```python
from build123d import *

# Parameters (mm, degrees)
SKETCH005_W    = 252
SKETCH005_H    = 268
PAD005_DEPTH   = 60
FILLET003_R    = 8
THICKNESS001_T = -3


with BuildPart() as part:
    # Sketch005 → Pad005 (new body)
    with BuildSketch(Plane.XY):
        with Locations((0, -134)):
            Rectangle(SKETCH005_W, SKETCH005_H)
    extrude(amount=PAD005_DEPTH)

    # Fillet003
    fillet003_edges = [part.edges().sort_by_distance(p)[0] for p in [
        (126, -268, 30),
        (-126, -268, 30),
    ]]
    fillet(fillet003_edges, radius=FILLET003_R)

    # Thickness001
    thickness001_openings = [part.faces().sort_by_distance(p)[0] for p in [
        (0, -133.946203, 60),
        (0, 0, 30),
        (0, -133.946203, 0),
    ]]
    offset(amount=THICKNESS001_T, openings=thickness001_openings)


solid = part.part
```
Input: part model. Units: mm. Frame: model coordinates. A direction names the side the tool comes from. Round coordinates to 2 decimals unless told otherwise and drop trailing zeros. Loops run counter-clockwise (first coordinate to the right, second up) from the corner with the lowest first, then second, coordinate; pieces in that order, holes last.
1) Section query C-C on x = -54.5. Return the cut outline in (y, z), plus the area to 3 significant figures.
Ans:
outline: (-268, 0) - (-265, 0) - (-265, 60) - (-268, 60) - close
area: 180 mm2
2) Material intervals for line 1 (X direction, y = -61, z = 19); line 2 (Y direction, x = -108, z = 42), sorted ascending.
Ans:
line 1: x = -126 to -123, 123 to 126
line 2: y = -268 to -265
3) Pin query (flat end, axial travel): pin 1 (8 mm diameter, centred on x = 89.5, z = 22, fed in from +Y). Return the tip coordinate at first contact, or that it passes through.
Ans:
pin 1: stops at y = -265
4) Section query A-A on y = -145.5. Return the cut outline in (x, z), plus the area to 3 significant figures.
Ans:
outline: (-126, 0) - (-123, 0) - (-123, 60) - (-126, 60) - close; (123, 0) - (126, 0) - (126, 60) - (123, 60) - close
area: 360 mm2
5) Section query B-B on z = 10.5. Return the cut outline in (x, y).
Ans:
outline: (-126, -260) arc R8 ccw to (-118, -268) - (118, -268) arc R8 ccw to (126, -260) - (126, 0) - (123, 0) - (123, -260) arc R5 cw to (118, -265) - (-118, -265) arc R5 cw to (-123, -260) - (-123, 0) - (-126, 0) - close
6) Set-up query: faces 1 (the flat face through (-2, -265, 30)), 2 (the cylindrical face through (-123.719, -265.594, 30.42)). Return all of +Z, -Z, +X, -X, +Y, -Y with unobstructed straight access to the full face (end or side cutting, diameter ignored); none if empty.
Ans:
face 1: +Z, -Z, +Y
face 2: +Z, -Z, -X, -Y
